from build123d import *

# Parameters (mm, degrees)
SKETCH_2_R          = 3
CUT_EXTRUDE_1_DEPTH = 4
SKETCH_3_R          = 2.5
CUT_EXTRUDE_2_DEPTH = 36


with BuildPart() as part:
    # 草图1 → 旋转1 (revolve)
    with BuildSketch(Plane.XY):
        with BuildLine():
            Line((20, 0), (35, 0))
            Line((35, 0), (35, 3))
            Line((35, 3), (24, 3))
            ThreePointArc((24, 3), (23.292893219, 3.292893219), (23, 4))
            Line((23, 4), (23, 9))
            ThreePointArc((23, 9), (22.707106781, 9.707106781), (22, 10))
            Line((22, 10), (14, 10))
            ThreePointArc((14, 10), (13.292893219, 10.292893219), (13, 11))
            Line((13, 11), (13, 49))
            Line((13, 49), (10, 49))
            Line((10, 49), (10, 7))
            Line((10, 7), (19, 7))
            ThreePointArc((19, 7), (19.707106781, 6.707106781), (20, 6))
            Line((20, 6), (20, 0))
        make_face()
    revolve(axis=Axis((0, 0, 0), (0, 1, 0)))

    # 草图2 → 切除-拉伸1 (cut, through all)
    with BuildSketch(Plane(origin=(0, 3, 0), x_dir=(1, 0, 0), z_dir=(0, 1, 0))):
        with Locations((0, 28.5)):
            Circle(SKETCH_2_R)
        with Locations((24.681724008, 14.25)):
            Circle(SKETCH_2_R)
        with Locations((24.681724008, -14.25)):
            Circle(SKETCH_2_R)
        with Locations((0, -28.5)):
            Circle(SKETCH_2_R)
        with Locations((-24.681724008, -14.25)):
            Circle(SKETCH_2_R)
        with Locations((-24.681724008, 14.25)):
            Circle(SKETCH_2_R)
    extrude(amount=-CUT_EXTRUDE_1_DEPTH, mode=Mode.SUBTRACT)

    # 草图3 → 切除-拉伸2 (cut, through all)
    with BuildSketch(Plane(origin=(0, 0, 0), x_dir=(0, 0, -1), z_dir=(1, 0, 0))):
        with Locations((0, 34)):
            Circle(SKETCH_3_R)
    extrude(amount=-CUT_EXTRUDE_2_DEPTH, mode=Mode.SUBTRACT)


solid = part.part
For this review, take the finished solid that the model builds, in its own axes (mm). A direction names the side the tool comes from. Coordinates: 2 decimals unless noted, no trailing zeros. Loops run counter-clockwise (first coordinate to the right, second up) from the corner with the lowest first, then second, coordinate; pieces in that order, holes last. Notation, with made-up numbers: (-36, 69) - (20, 69) arc R10 ccw to (20, 83) - close; hole circle Ø9 at (30.25, -10). An arc over 180 degrees is marked (long way). Use a Markdown table: item, result. Add a question column.
Item 1: We need section B-B (z = -28.5). Give the boundary of the cut face in (x, y), and give its area (3 significant figures).
Item 2: Mouldability with a two-part tool opening along X and no side actions: class faces 1 (the face through (-23.297, 1.521, -11.588)), 2 (the face through (-28, 2, 21)), 3 (the face through (7, 49, 8)) as pulls with the +X half, pulls with the -X half, needs draft (parallel to the pull), parting line crosses it, or undercut.
Item 3: Insertion check: pin 1 Ø19 at (x, z) = (8.5, -0.5) entering from -Y; pin 2 Ø9.5 at (x, z) = (24.68, 14.25) entering from +Y; pin 3 Ø10 at (y, z) = (25, 14.5) entering from -X. Each pin has a flat end and moves straight along its axis. Give the tip position at first contact, or say it passes through.
Item 4: We need section C-C (y = 27). Give the boundary of the cut face in (x, z).
Item 5: We need section A-A (z = 0). Give the number of separate pieces and of enclosed holes in the cut face, and give its area (3 significant figures).
Item 6: We need section D-D (x = 30). Give the boundary of the cut face in (y, z).
Item 7: For line 1 (Z direction, x = 0, y = 1); line 2 (X direction, y = 2, z = -13.5); line 3 (X direction, y = 1, z = 14), list the stretches that pass through material, from the lowest coordinate up.
Item 8: Tool access review of faces 4 (the face through (-4.336, 2.958, 19.524)), 5 (the face through (-11.3, 32.5, 2)), 6 (the face through (-23.297, 1.521, 16.912)), 7 (the face through (-2.994, 6.535, -22.804)), 8 (the face through (-15, 0, 15)): name each direction out of +Z, -Z, +X, -X, +Y, -Y from which nothing blocks a thin tool from reaching the whole face with its end or side.
Results list:
| question | item | result |
|---|---|---|
| 1 | outline | (-20.32, 0) - (-3, 0) - (-3, 3) - (-20.32, 3) - close; (3, 0) - (20.32, 0) - (20.32, 3) - (3, 3) - close |
| 1 | area | 104 mm^2 |
| 2 | face 1 | undercut |
| 2 | face 2 | parting line crosses it |
| 2 | face 3 | needs draft |
| 3 | pin 1 | stops at y = 7 |
| 3 | pin 2 | stops at y = 3.03 |
| 3 | pin 3 | stops at x = -8.87 |
| 4 | outline | circle Ø26 at (0, 0); hole circle Ø20 at (0, 0) |
| 5 | separate pieces | 3 |
| 5 | enclosed holes | 0 |
| 5 | area | 412 mm^2 |
| 6 | outline | (0, -18.03) - (3, -18.03) - (3, 18.03) - (0, 18.03) - close |
| 7 | line 1 | z = -35 to -31.5, -25.5 to -20, 20 to 25.5, 31.5 to 35 |
| 7 | line 2 | x = -32.29 to -27.59, -21.78 to -14.76, 14.76 to 21.78, 27.59 to 32.29 |
| 7 | line 3 | x = -32.08 to -27.67, -21.69 to -14.28, 14.28 to 21.69, 27.67 to 32.08 |
| 8 | face 4 | -Y |
| 8 | face 5 | -X |
| 8 | face 6 | +Y, -Y |
| 8 | face 7 | +Y |
| 8 | face 8 | +Z, -Z, +X, -X, -Y |
